from build123d import *

# Parameters (mm, degrees)
BOX023_W               = 100
BOX023_H               = 100
BOX023_DEPTH           = 30
BOX023_PLACEMENT_ANGLE = -45
BOX022_W               = 30
BOX022_H               = 100
BOX022_DEPTH           = 30
BOX022_PLACEMENT_ANGLE = -45
PAD001_DEPTH           = 501


with BuildPart() as cube008:
    # Box023 → Box023 (new body)
    with BuildSketch(Plane.XY):
        with Locations((50, 50)):
            Rectangle(BOX023_W, BOX023_H)
    extrude(amount=BOX023_DEPTH)


with BuildPart() as cube008_1:
    # Box023 placement: moved
    add(cube008.part.moved(Location((-3, 498, -3))).rotate(Axis((-3, 498, -3), (0, 0, 1)), BOX023_PLACEMENT_ANGLE))


with BuildPart() as cube007:
    # Box022 → Box022 (new body)
    with BuildSketch(Plane.XY):
        with Locations((15, 50)):
            Rectangle(BOX022_W, BOX022_H)
    extrude(amount=BOX022_DEPTH)


with BuildPart() as cube007_1:
    # Box022 placement: moved
    add(cube007.part.moved(Location((-3, -3, -3))).rotate(Axis((-3, -3, -3), (0, 0, 1)), BOX022_PLACEMENT_ANGLE))


with BuildPart() as rahmen3:
    # Sketch001 → Pad001 (new body)
    with BuildSketch(Plane.XZ.offset(3)):
        Polygon((0, 17), (0, 0), (27, 0), (27, -3), (-3, -3), (-3, 17), align=None)
    extrude(amount=-PAD001_DEPTH)

    # Cut003: cut Cube007
    add(cube007_1.part, mode=Mode.SUBTRACT)

    # Cut004: cut Cube008
    add(cube008_1.part, mode=Mode.SUBTRACT)


solid = rahmen3.part
Could you check a few things on this model? Use its own coordinates, in mm. A direction names the side the tool comes from. Coordinates: 2 decimals unless noted, no trailing zeros. Order: outer loops, then holes, each group sorted by start corner. A loop starts at its lowest first (then second) coordinate and runs counter-clockwise, first axis right, second up.
Q1. Please list where these lines run through material, in increasing order: L1, parallel to Z at x = 1.5, y = 414; L2, parallel to Y at x = 18, z = -1.
Q2. Suppose I cut it at B-B on x = 14.5. Please give me the cut outline in (y, z), and give its area (3 significant figures).
Q3. Will these pins go through, and if not, where does the flat tip stop? pin 1 (12 mm diameter, centred on y = 187, z = 12.5, fed in from +X); pin 2 (10 mm diameter, centred on x = 14, z = 2.5, fed in from +Y).
Q4. Suppose I cut it at C-C on z = 12.5. Please give me the cut outline in (x, y), and give its area (3 significant figures).
Q5. Suppose I cut it at A-A on y = 286. Please give me the cut outline in (x, z), and give its area (3 significant figures).
Q6. Which directions (+Z, -Z, +X, -X, +Y, -Y) give clear straight access to the entire face, cutting with the end or side of a thin tool? Please do faces 1 (the flat face through (-3, 244, 7)), 2 (the flat face through (13, 244, 0)).
Answer:
1. L1: z = -3 to 0
1. L2: y = 18 to 477
2. outline: (14.5, -3) - (480.5, -3) - (480.5, 0) - (14.5, 0) - close
2. area: 1,400 mm2
3. pin 1: stops at x = 0
3. pin 2: stops at y = 485.33
4. outline: (-3, -3) - (0, 0) - (0, 495) - (-3, 498) - close
4. area: 1,490 mm2
5. outline: (-3, -3) - (27, -3) - (27, 0) - (0, 0) - (0, 17) - (-3, 17) - close
5. area: 141 mm2
6. face 1: +Z, -Z, -X, +Y, -Y
6. face 2: +Z, +X, +Y, -Y
